The listing builds one solid part. Answer for the finished solid, in the listing's coordinates (mm). Round coordinates to 2 decimals unless told otherwise and drop trailing zeros. Write each loop counter-clockwise with the first axis right and the second up, starting at its lowest first coordinate (ties: lowest second). Pieces come first, ordered by that corner, then holes.
(1) A cutting plane is placed at B-B, the plane z = -606. Give the vertices of the cut face in (x, y).
(2) A cutting plane is placed at A-A, the plane y = 12. Give the vertices of the cut face in (x, z), and give its area (3 significant figures).
(3) Find the intervals of material crossed by probe 1 along X at (y, z) = (68.25, 500); probe 2 along X at (y, z) = (22, 190.5); probe 3 along Z at (x, y) = (36, 67.5), in increasing order.
(4) Each of these flat-tipped pins is pushed along its axis until it touches: pin 1 Ø10 at (y, z) = (24, 183.5) entering from -X; pin 2 Ø19 at (x, z) = (35, -170) entering from -Y; pin 3 Ø8 at (y, z) = (17.5, -159) entering from +X; pin 4 Ø3 at (x, y) = (28.5, 61) entering from -Z. Where does it stop, or does it pass through?
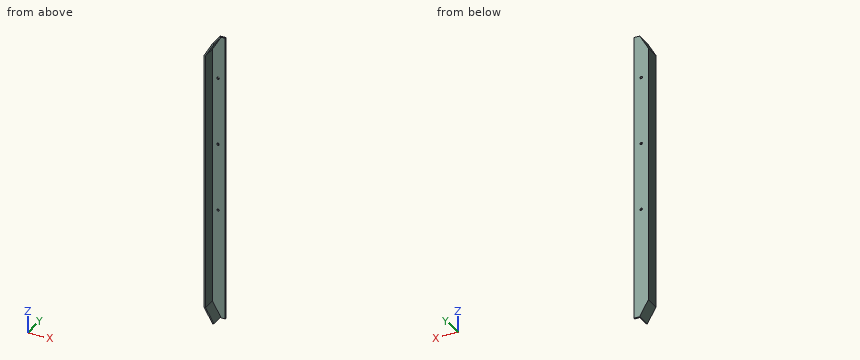
from build123d import *

# Parameters (mm, degrees)
BOSS_EXTRUDE1_DEPTH     = 640
BOSS_EXTRUDE2_DEPTH     = 63
BOSS_EXTRUDE3_DEPTH     = 7
CUT_EXTRUDE1_DEPTH      = 10
CUT_EXTRUDE1_DEPTH_BACK = 10
SKETCH28_R              = 6


with BuildPart() as part:
    # Sketch1 → Boss-Extrude1 (new body)
    with BuildSketch(Plane.XY):
        Polygon((0, 0), (0, 70), (70, 70), (70, 63), (7, 63), (7, 0), align=None)
    extrude(amount=BOSS_EXTRUDE1_DEPTH)

    # Sketch23 → Boss-Extrude2 (add)
    with BuildSketch(Plane(origin=(0, 0, 0), x_dir=(1, 0, 0), z_dir=(0, 1, 0))):
        Polygon((0, -640), (42.5, -713.612159322), (48.562177826, -710.112159322), (7, -640), align=None)
    extrude(amount=BOSS_EXTRUDE2_DEPTH)

    # Sketch25 → Boss-Extrude3 (add)
    with BuildSketch(Plane(origin=(0, 63, 0), x_dir=(1, 0, 0), z_dir=(0, 1, 0))):
        Polygon((70, -640), (0, -640), (42.5, -713.612159322), (70, -713.612159322), align=None)
    extrude(amount=BOSS_EXTRUDE3_DEPTH)

    # Mirror1: part across plane


with BuildPart() as part_1:
    add(part.part)
    add(part.part.mirror(Plane.XY))

    # Sketch28 → Cut-Extrude1 (cut, two sides: drawn at the far end of the back side and taken through both)
    with BuildSketch(Plane(origin=(0, 70, 0), x_dir=(1, 0, 0), z_dir=(0, 1, 0)).offset(-CUT_EXTRUDE1_DEPTH_BACK)):
        with Locations(Location((35, -500, 0), (0, 0, 90))):
            Circle(SKETCH28_R)
        with Locations(Location((35, -165, 0), (0, 0, 90))):
            Circle(SKETCH28_R)
        with Locations(Location((35, 170, 0), (0, 0, 90))):
            Circle(SKETCH28_R)
    extrude(amount=CUT_EXTRUDE1_DEPTH + CUT_EXTRUDE1_DEPTH_BACK, mode=Mode.SUBTRACT)


solid = part_1.part
Solutions:
1. outline: (0, 0) - (7, 0) - (7, 63) - (70, 63) - (70, 70) - (0, 70) - close
2. outline: (0, -640) - (42.5, -713.61) - (48.56, -710.11) - (7, -640) - (7, 640) - (48.56, 710.11) - (42.5, 713.61) - (0, 640) - close
2. area: 10,000 mm2
3. probe 1: x = 0 to 29, 41 to 70
3. probe 2: x = 0 to 7
3. probe 3: z = -702.35 to -175.92, -164.08 to 159.08, 170.92 to 494.08, 505.92 to 702.35
4. pin 1: stops at x = 0
4. pin 2: stops at y = 63
4. pin 3: stops at x = 7
4. pin 4: stops at z = -691.96
